The model under review builds one solid part; all positions refer to its coordinate system, in mm. A direction names the side the tool comes from. Coordinates: 2 decimals unless noted, no trailing zeros. Write each loop counter-clockwise with the first axis right and the second up, starting at its lowest first coordinate (ties: lowest second). Pieces come first, ordered by that corner, then holes.
1) Mouldability with a two-part tool opening along Z and no side actions: class faces 1 (the cylindrical face through (2.343, 17.847, -0.493)), 2 (the flat face through (0, 0, -7.5)), 3 (the flat face through (0, 0, -2)), 4 (the cylindrical face through (-4.01, -18.06, 1.97)) as released by +Z, released by -Z, zero draft, split by the parting line, or undercut.
2) Add section C-C, the plane y = 0. State the section outline as (x, z) points, then the cut area to 3 significant figures.
3) Machinability: for faces 5 (the flat face through (0, 1, 1)), 6 (the cylindrical face through (-9.139, 14.334, -5.493)), 7 (the cylindrical face through (4.01, -18.06, -2.97)), 8 (the cylindrical face through (3, 0, -9)), which of the approach directions +Z, -Z, +X, -X, +Y, -Y give a long, thin tool a straight path to every point of the face, cutting with its end or side? Answer none if there is none.
4) Add section D-D, the plane x = 12. State the section outline as (y, z) points.
5) For P1, Ø6, axis at x = 4.5, z = -5.5, coming from the -Y side; P2, Ø0.7, axis at x = -0.5, z = 0, coming from the -Y side; P3, Ø0.8, axis at x = 0.5, y = 0, coming from the +Z side, all flat-tipped, find the tip position at first contact; note any pin that passes through.
6) Add section B-B, the plane z = -8.25. State the section outline as (x, y) points.
7) Add section A-A, the plane x = 0. State the section outline as (y, z) points.
8) For line 1 (Z direction, x = -11, y = 14); line 2 (Y direction, x = 0, z = -9.1); line 3 (Y direction, x = 0, z = 0.4), list the stretches that pass through material, from the lowest coordinate up.
from build123d import *

# Parameters (mm, degrees)
SKETCH_1_R          = 18.5
EXTRUDE_1_DEPTH     = 4
SKETCH_2_R          = 18
EXTRUDE_2_DEPTH     = 1
SKETCH_3_R          = 18.5
EXTRUDE_3_DEPTH     = 4
SKETCH_4_R          = 17
EXTRUDE_4_DEPTH     = 1
SKETCH_5_R          = 18.5
EXTRUDE_5_DEPTH     = 4
CUT_EXTRUDE_1_DEPTH = 6
SKETCH_7_R          = 3
CUT_EXTRUDE_2_DEPTH = 2.5


with BuildPart() as part:
    # 草图1 → 凸台-拉伸1 (new body)
    with BuildSketch(Plane.XY):
        Circle(SKETCH_1_R)
    extrude(amount=EXTRUDE_1_DEPTH)

    # 草图2 → 凸台-拉伸2 (add)
    with BuildSketch(Plane(origin=(0, 0, 0), x_dir=(-1, 0, 0), z_dir=(0, 0, -1))):
        Circle(SKETCH_2_R)
    extrude(amount=EXTRUDE_2_DEPTH)

    # 草图3 → 凸台-拉伸3 (add)
    with BuildSketch(Plane(origin=(0, 0, -1), x_dir=(-1, 0, 0), z_dir=(0, 0, -1))):
        Circle(SKETCH_3_R)
    extrude(amount=EXTRUDE_3_DEPTH)

    # 草图4 → 凸台-拉伸4 (add)
    with BuildSketch(Plane(origin=(0, 0, -5), x_dir=(-1, 0, 0), z_dir=(0, 0, -1))):
        Circle(SKETCH_4_R)
    extrude(amount=EXTRUDE_4_DEPTH)

    # 草图5 → 凸台-拉伸5 (add)
    with BuildSketch(Plane(origin=(0, 0, -6), x_dir=(-1, 0, 0), z_dir=(0, 0, -1))):
        Circle(SKETCH_5_R)
    extrude(amount=EXTRUDE_5_DEPTH)

    # 草图6 → 切除-拉伸1 (cut)
    with BuildSketch(Plane.XY.offset(4)):
        with BuildLine():
            Line((1.118033989, 1), (-1.118033989, 1))
            ThreePointArc((-1.118033989, 1), (0, -1.5), (1.118033989, 1))
        make_face()
    extrude(amount=-CUT_EXTRUDE_1_DEPTH, mode=Mode.SUBTRACT)

    # 草图7 → 切除-拉伸2 (cut)
    with BuildSketch(Plane(origin=(0, 0, -10), x_dir=(-1, 0, 0), z_dir=(0, 0, -1))):
        Circle(SKETCH_7_R)
    extrude(amount=-CUT_EXTRUDE_2_DEPTH, mode=Mode.SUBTRACT)


solid = part.part
Geometry results:
1. face 1: undercut
1. face 2: released by -Z
1. face 3: released by +Z
1. face 4: zero draft
2. outline: (-18.5, -10) - (-3, -10) - (-3, -7.5) - (3, -7.5) - (3, -10) - (18.5, -10) - (18.5, -6) - (17, -6) - (17, -5) - (18.5, -5) - (18.5, -1) - (18, -1) - (18, 0) - (18.5, 0) - (18.5, 4) - (1.5, 4) - (1.5, -2) - (-1.5, -2) - (-1.5, 4) - (-18.5, 4) - (-18.5, 0) - (-18, 0) - (-18, -1) - (-18.5, -1) - (-18.5, -5) - (-17, -5) - (-17, -6) - (-18.5, -6) - close
2. area: 481 mm2
3. face 5: +Z
3. face 6: none
3. face 7: +Z, -Z
3. face 8: -Z
4. outline: (-14.08, -10) - (14.08, -10) - (14.08, -6) - (12.04, -6) - (12.04, -5) - (14.08, -5) - (14.08, -1) - (13.42, -1) - (13.42, 0) - (14.08, 0) - (14.08, 4) - (-14.08, 4) - (-14.08, 0) - (-13.42, 0) - (-13.42, -1) - (-14.08, -1) - (-14.08, -5) - (-12.04, -5) - (-12.04, -6) - (-14.08, -6) - close
5. P1: stops at y = -18.44
5. P2: stops at y = -18.5
5. P3: stops at z = -2
6. outline: circle Ø37 at (0, 0); hole circle Ø6 at (0, 0)
7. outline: (-18.5, -10) - (-3, -10) - (-3, -7.5) - (3, -7.5) - (3, -10) - (18.5, -10) - (18.5, -6) - (17, -6) - (17, -5) - (18.5, -5) - (18.5, -1) - (18, -1) - (18, 0) - (18.5, 0) - (18.5, 4) - (1, 4) - (1, -2) - (-1.5, -2) - (-1.5, 4) - (-18.5, 4) - (-18.5, 0) - (-18, 0) - (-18, -1) - (-18.5, -1) - (-18.5, -5) - (-17, -5) - (-17, -6) - (-18.5, -6) - close
8. line 1: z = -10 to -6, -5 to 4
8. line 2: y = -18.5 to -3, 3 to 18.5
8. line 3: y = -18.5 to -1.5, 1 to 18.5
